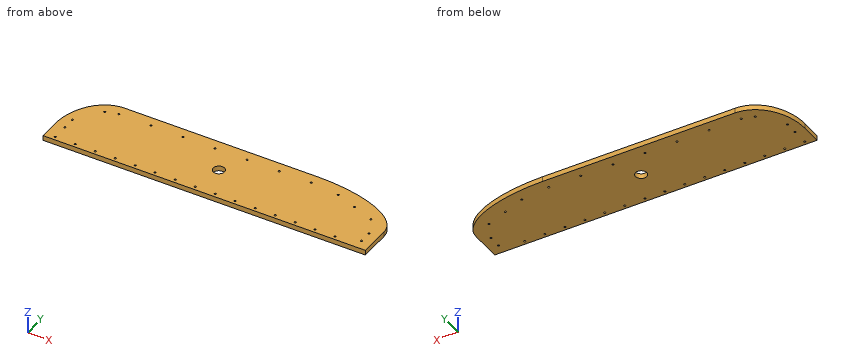
```python
from build123d import *

# Parameters (mm, degrees)
BOSS_EXTRUDE1_DEPTH = 12.7
SKETCH12_R          = 2.38125
CUT_EXTRUDE10_DEPTH = 839.320256645
SKETCH13_R          = 2.413
CUT_EXTRUDE11_DEPTH = 839.320256645
LPATTERN1_COUNT     = 15
LPATTERN1_PITCH     = 50.8
SKETCH17_R          = 14.2875
CUT_EXTRUDE15_DEPTH = 839.320256645


with BuildPart() as part:
    # Sketch1 → Boss-Extrude1 (new body)
    with BuildSketch(Plane.XY):
        with BuildLine():
            Line((0, 0), (819.15, 0))
            Line((819.15, 0), (819.15, 79.375))
            add(Edge.make_bspline(
                [(819.15, 79.375), (819.15, 177.8), (590.55, 177.8)],
                knots=[0, 0, 0, 1.570796327, 1.570796327, 1.570796327], degree=2, weights=[1, 0.707106781, 1]))
            Line((590.55, 177.8), (101.6, 177.8))
            add(Edge.make_bspline(
                [(101.6, 177.8), (0, 177.8), (0, 50.8)],
                knots=[3.141592654, 3.141592654, 3.141592654, 4.71238898, 4.71238898, 4.71238898], degree=2, weights=[1, 0.707106781, 1]))
            Line((0, 50.8), (0, 0))
        make_face()
    extrude(amount=BOSS_EXTRUDE1_DEPTH)

    # Sketch12 → Cut-Extrude10 (cut, through all)
    with BuildSketch(Plane.XY.offset(12.7)):
        with Locations((25.4, 50.8)):
            Circle(SKETCH12_R)
        with Locations((346.075, 152.4)):
            Circle(SKETCH12_R)
        with Locations((264.583333333, 152.4)):
            Circle(SKETCH12_R)
        with Locations((101.6, 152.4)):
            Circle(SKETCH12_R)
        with Locations((183.091666667, 152.4)):
            Circle(SKETCH12_R)
        with Locations((71.12, 143.51)):
            Circle(SKETCH12_R)
        with Locations((25.4, 82.55)):
            Circle(SKETCH12_R)
        with Locations(Location((509.058333333, 152.4, 0), (0, 0, 180))):
            Circle(SKETCH12_R)
        with Locations(Location((590.55, 152.4, 0), (0, 0, 180))):
            Circle(SKETCH12_R)
        with Locations(Location((427.566666667, 152.4, 0), (0, 0, 180))):
            Circle(SKETCH12_R)
        with Locations((793.75, 57.15)):
            Circle(SKETCH12_R)
        with Locations((793.75, 25.4)):
            Circle(SKETCH12_R)
        with Locations((717.55, 123.825)):
            Circle(SKETCH12_R)
        with Locations((664.038787502, 143.891704687)):
            Circle(SKETCH12_R)
        with Locations((771.061212498, 103.758295313)):
            Circle(SKETCH12_R)
    extrude(amount=-CUT_EXTRUDE10_DEPTH, mode=Mode.SUBTRACT)

    # Sketch13 → Cut-Extrude11 (cut, through all)
    with BuildSketch(Plane.XY.offset(12.7)):
        with Locations((25.4, 9.525)):
            Circle(SKETCH13_R)
    cut_extrude11 = extrude(amount=-CUT_EXTRUDE11_DEPTH, mode=Mode.SUBTRACT)

    # LPattern1: Cut-Extrude11 ×15
    with Locations(*[(i * LPATTERN1_PITCH, 0, 0) for i in range(1, LPATTERN1_COUNT)]):
        add(cut_extrude11, mode=Mode.SUBTRACT)

    # Sketch17 → Cut-Extrude15 (cut, through all)
    with BuildSketch(Plane.XY.offset(12.7)):
        with Locations((393.7, 88.9)):
            Circle(SKETCH17_R)
    extrude(amount=-CUT_EXTRUDE15_DEPTH, mode=Mode.SUBTRACT)


solid = part.part
```
Input: part model. Units: mm. Frame: model coordinates. Give positions to 0.01 mm unless a question says otherwise; leave off trailing zeros. Order: outer loops, then holes, each group sorted by start corner. A loop starts at its lowest first (then second) coordinate and runs counter-clockwise, first axis right, second up. Notation, with made-up numbers: M 22,76 L 50,76 A28 ccw 50,104 Z; hole C -18.5,49.25 d2. An arc over 180 degrees is marked long. Return JSON: item names as keys, results as strings.
Item 1: Cut plane A-A (x = 393.7). Return loops of the section in (y, z), then the cut area to 3 significant figures.
Solutions:
{"outline": "M 0,0 L 74.61,0 L 74.61,12.7 L 0,12.7 Z; M 103.19,0 L 177.8,0 L 177.8,12.7 L 103.19,12.7 Z", "area": "1,900 mm^2"}
Item 2: Cut plane B-B (z = 5.75). State how many separate pieces and enclosed holes the cut face has, then the cut area to 3 significant figures.
Solutions:
{"separate pieces": "1", "enclosed holes": "31", "area": "137,000 mm^2"}
Item 3: First-contact query: P1, Ø2, axis at y = 128, z = 4, coming from the -X side. Flat tip, straight axial feed; report the tip coordinate or a pass-through.
Solutions:
{"P1": "x = 20.32"}
Item 4: Ray query, probe 1 along Y at (x, z) = (228.6, 6); probe 2 along Y at (x, z) = (393.7, 5.75); probe 3 along X at (y, z) = (143.51, 4). Return the intervals inside material, ascending.
Solutions:
{"probe 1": "0 to 7.11, 11.94 to 177.8", "probe 2": "0 to 74.61, 103.19 to 177.8", "probe 3": "32.16 to 68.74, 73.5 to 661.69, 666.39 to 763.95"}
